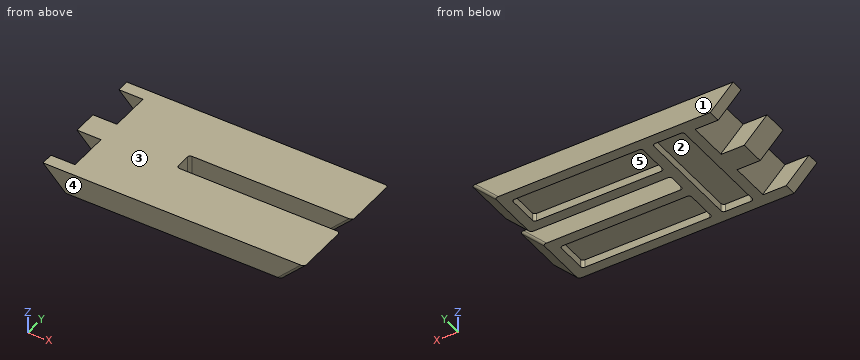
from build123d import *

# Parameters (mm, degrees)
BOSS_EXTRUDE1_DEPTH = 3.5
CUT_EXTRUDE1_DEPTH  = 29.5
CUT_EXTRUDE2_DEPTH  = 29.5
CAVITY1_START       = -8
CAVITY1_DEPTH       = 6
CAVITY1_START_2     = 2
CAVITY1_2_DEPTH     = 6
SKETCH4_W           = 4.949747468
SKETCH4_H           = 6
CUT_EXTRUDE3_DEPTH  = 0.1
CUT_EXTRUDE4_DEPTH  = 0.1
CUT_EXTRUDE5_DEPTH  = 0.1
CUT_EXTRUDE6_DEPTH  = 0.1
CUT_EXTRUDE7_DEPTH  = 0.1
SKETCH9_W           = 19.9
SKETCH9_H           = 5.3
SKETCH9_W_2         = 4.764466094
SKETCH9_H_2         = 16.8
CUT_EXTRUDE8_DEPTH  = 1.2
FILLET1_R           = 0.4


# Read off the part's stored shape, not the designer's step: Cavity1
with BuildPart() as part:
    # Sketch1 → Boss-Extrude1 (new body)
    with BuildSketch(Plane.XY):
        Polygon((20, -1.5), (20, -10), (-20, -10), (-20, 10), (20, 10), (20, 1.5), (-5, 1.5), (-5, -1.5), align=None)
    extrude(amount=BOSS_EXTRUDE1_DEPTH)

    # Sketch2 → Cut-Extrude1 (cut, through all)
    with BuildSketch(Plane(origin=(0, 10, 0), x_dir=(1, 0, 0), z_dir=(0, 1, 0))):
        Polygon((20, -3.5), (16.5, 0), (20, 0), align=None)
    extrude(amount=-CUT_EXTRUDE1_DEPTH, mode=Mode.SUBTRACT)

    # Sketch3 → Cut-Extrude2 (cut, through all)
    with BuildSketch(Plane(origin=(0, 10, 0), x_dir=(1, 0, 0), z_dir=(0, 1, 0))):
        Polygon((-20, -3.5), (-16.5, 0), (-20, 0), align=None)
    extrude(amount=-CUT_EXTRUDE2_DEPTH, mode=Mode.SUBTRACT)

    # Cavity1 outline → Cavity1 (cut)
    with BuildSketch(Plane(origin=(0, 0, 0), x_dir=(1, 0, 0), z_dir=(0, 1, 0)).offset(CAVITY1_START)):
        Polygon((-16.464466094, -3.5), (-12.964466094, 0), (-16.5, 0), (-20, -3.5), align=None)
    extrude(amount=CAVITY1_DEPTH, mode=Mode.SUBTRACT)

    # Cavity1 2 outline → Cavity1 2 (cut)
    with BuildSketch(Plane(origin=(0, 0, 0), x_dir=(1, 0, 0), z_dir=(0, 1, 0)).offset(CAVITY1_START_2)):
        Polygon((-16.464466094, -3.5), (-12.964466094, 0), (-16.5, 0), (-20, -3.5), align=None)
    extrude(amount=CAVITY1_2_DEPTH, mode=Mode.SUBTRACT)

    # Sketch4 → Cut-Extrude3 (cut)
    with BuildSketch(Plane(origin=(-6.482233047, 0, -6.482233047), x_dir=(-0.7071067811865464, 0, 0.7071067811865488), z_dir=(-0.7071067811865488, 0, -0.7071067811865464))):
        with Locations((11.642135624, -5)):
            Rectangle(SKETCH4_W, SKETCH4_H)
        with Locations((11.642135624, 5)):
            Rectangle(SKETCH4_W, SKETCH4_H)
    extrude(amount=-CUT_EXTRUDE3_DEPTH, mode=Mode.SUBTRACT)

    # Sketch5 → Cut-Extrude4 (cut)
    with BuildSketch(Plane.XZ.offset(2)):
        Polygon((-16.5, 0), (-12.964466094, 0), (-12.893755416, 0.070710678), (-16.323044738, 3.5), (-20, 3.5), align=None)
    extrude(amount=-CUT_EXTRUDE4_DEPTH, mode=Mode.SUBTRACT)

    # Sketch6 → Cut-Extrude5 (cut)
    with BuildSketch(Plane.XZ.offset(-8)):
        Polygon((-16.323044738, 3.5), (-20, 3.5), (-16.5, 0), (-12.964466094, 0), (-12.893755416, 0.070710678), align=None)
    extrude(amount=-CUT_EXTRUDE5_DEPTH, mode=Mode.SUBTRACT)

    # Sketch7 → Cut-Extrude6 (cut)
    with BuildSketch(Plane(origin=(0, 2, 0), x_dir=(1, 0, 0), z_dir=(0, 1, 0))):
        Polygon((-20, -3.5), (-16.323044738, -3.5), (-12.893755416, -0.070710678), (-12.964466094, 0), (-16.5, 0), align=None)
    extrude(amount=-CUT_EXTRUDE6_DEPTH, mode=Mode.SUBTRACT)

    # Sketch8 → Cut-Extrude7 (cut)
    with BuildSketch(Plane(origin=(0, -8, 0), x_dir=(1, 0, 0), z_dir=(0, 1, 0))):
        Polygon((-20, -3.5), (-16.323044738, -3.5), (-12.893755416, -0.070710678), (-12.964466094, 0), (-16.5, 0), align=None)
    extrude(amount=-CUT_EXTRUDE7_DEPTH, mode=Mode.SUBTRACT)

    # Sketch9 → Cut-Extrude8 (cut)
    with BuildSketch(Plane(origin=(0, 0, 0), x_dir=(-1, 0, 0), z_dir=(0, 0, -1))):
        with Locations((-4.95, 5.75)):
            Rectangle(SKETCH9_W, SKETCH9_H)
        with Locations((-4.95, -5.75)):
            Rectangle(SKETCH9_W, SKETCH9_H)
        with Locations((8.982233047, 0)):
            Rectangle(SKETCH9_W_2, SKETCH9_H_2)
    extrude(amount=-CUT_EXTRUDE8_DEPTH, mode=Mode.SUBTRACT)

    # Fillet1
    fillet1_edges = [part.edges().sort_by_distance(p)[0] for p in [
        (-5, 1.5, 1.75),
        (-5, -1.5, 1.75),
        (-6.6, -8.4, 0.6),
        (-6.6, 8.4, 0.6),
        (-11.364466094, 8.4, 0.6),
        (-11.364466094, -8.4, 0.6),
        (14.9, -8.4, 0.6),
        (14.9, -3.1, 0.6),
        (-5, -3.1, 0.6),
        (-5, -8.4, 0.6),
        (14.9, 3.1, 0.6),
        (14.9, 8.4, 0.6),
        (-5, 8.4, 0.6),
        (-5, 3.1, 0.6),
        (18.25, -1.5, 1.75),
        (18.25, -10, 1.75),
        (18.25, 1.5, 1.75),
        (18.25, 10, 1.75),
    ]]
    fillet(fillet1_edges, radius=FILLET1_R)


solid = part.part
Work out the finished part from the listing and answer in its coordinate system (mm). Face numbers are marked on the shaded views. A direction names the side the tool comes from. Round coordinates to 2 decimals unless told otherwise and drop trailing zeros. Loops run counter-clockwise (first coordinate to the right, second up) from the corner with the lowest first, then second, coordinate; pieces in that order, holes last. Notation, with made-up numbers: (38.5, 53) - (76.5, 53) arc R30 ccw to (76.5, 81) - close; hole circle Ø2 at (84, 74.5). An arc over 180 degrees is marked (long way). Use one line per item in the form item = value. Start each with the question number.
(1) Find section C-C on x = -8.5. Determine the outline of the cut face in (y, z).
(2) Determine the mould class of the marked faces 3, 4 and 5 for opening direction Y: +Y half, -Y half, draft (parallel to the pull), parting line (faces both ways), or undercut.
(3) Consider line 1 (Y direction, x = 13.5, z = 0.55); line 2 (Y direction, x = -16, z = 1); line 3 (Y direction, x = -1, z = 1.25). Determine where each line is inside the solid, lowest interval first.
(4) Which of the six approach directions +Z, -Z, +X, -X, +Y, -Y give full straight-line access (tool end or side, diameter ignored) to the marked faces 1 and 2?
(5) Find section D-D on z = 0.6. Give the number of separate pieces and of enclosed holes in the cut face, and give its area (3 significant figures).
(6) Flat-ended cylindrical pins translate along their axes: P1, Ø1, axis at y = -6.5, z = 0.5, coming from the -X side; P2, Ø2, axis at y = -2.5, z = 2, coming from the -X side; P3, Ø0.6, axis at y = 7, z = 1, coming from the -X side. Find the tip coordinate at first contact, or state that the pin passes through.
(7) Find section B-B on y = 5.5. Determine the outline of the cut face in (x, z).
(8) Find section A-A on x = 9. Determine the outline of the cut face in (y, z).
Answer list:
q1.outline = (-10, 0) - (-8.4, 0) - (-8.4, 1.2) - (8.4, 1.2) - (8.4, 0) - (10, 0) - (10, 3.5) - (-10, 3.5) - close
q2.face_3 = draft
q2.face_4 = -Y half
q2.face_5 = undercut
q3.line_1 = -10 to -8.4, -3.1 to -1.5, 1.5 to 3.1, 8.4 to 10
q3.line_2 = -10 to -8.1, -1.9 to 1.9, 8.1 to 10
q3.line_3 = -10 to -1.5, 1.5 to 10
q4.face_1 = +Z, -Z, +X, -X, +Y
q4.face_2 = -Z
q5.separate_pieces = 1
q5.enclosed_holes = 3
q5.area = 281 mm^2
q6.P1 = -13.82
q6.P2 = -19.3
q6.P3 = -14.12
q7.outline = (-16.32, 3.5) - (-12.89, 0.07) - (-12.96, 0) - (-11.36, 0) - (-11.36, 1.2) - (-6.6, 1.2) - (-6.6, 0) - (-5, 0) - (-5, 1.2) - (14.9, 1.2) - (14.9, 0) - (16.5, 0) - (20, 3.5) - close
q8.outline = (-10, 0) - (-8.4, 0) - (-8.4, 1.2) - (-3.1, 1.2) - (-3.1, 0) - (-1.5, 0) - (-1.5, 3.5) - (-10, 3.5) - close; (1.5, 0) - (3.1, 0) - (3.1, 1.2) - (8.4, 1.2) - (8.4, 0) - (10, 0) - (10, 3.5) - (1.5, 3.5) - close
